Read the model definition and answer for the solid it produces. Units are mm, in the model's axes. Face numbers are marked on the shaded views. Coordinates: 2 decimals unless noted, no trailing zeros. Loops run counter-clockwise (first coordinate to the right, second up) from the corner with the lowest first, then second, coordinate; pieces in that order, holes last.
from build123d import *

# Parameters (mm, degrees)
SKETCH2_R               = 50
SKETCH2_R_2             = 25
BOSS_EXTRUDE1_DEPTH     = 10
CUT_EXTRUDE1_DEPTH      = 72.414284285
CUT_EXTRUDE1_DEPTH_BACK = 72.414284285
SKETCH3_R               = 1.5
SKETCH5_W               = 42.1
SKETCH5_H               = 42.1
SKETCH5_W_2             = 28.1
SKETCH5_H_2             = 28.1
BOSS_EXTRUDE3_DEPTH     = 32
SKETCH6_W               = 15
SKETCH6_H               = 10
CUT_EXTRUDE2_DEPTH      = 7
SKETCH7_W               = 42.1
SKETCH7_H               = 42.1
SKETCH7_R               = 14.05
BOSS_EXTRUDE4_DEPTH     = 40
CUT_EXTRUDE3_START      = -72
CUT_EXTRUDE3_DEPTH      = 72
CIRPATTERN1_COUNT       = 4
SKETCH12_R              = 21.05
SKETCH12_W              = 20.1
SKETCH12_H              = 20.1
BOSS_EXTRUDE5_DEPTH     = 10


with BuildPart() as part:
    # Sketch2 → Boss-Extrude1 (new body)
    with BuildSketch(Plane.XY):
        Circle(SKETCH2_R)
        Circle(SKETCH2_R_2, mode=Mode.SUBTRACT)
    extrude(amount=BOSS_EXTRUDE1_DEPTH)

    # Sketch3 → Cut-Extrude1 (cut, two sides: drawn at the far end of the back side and taken through both)
    with BuildSketch(Plane(origin=(0, 0, 0), x_dir=(1, 0, 0), z_dir=(0, 1, 0)).offset(-CUT_EXTRUDE1_DEPTH_BACK)):
        with Locations(Location((0, -5, 0), (0, 0, 270))):
            Circle(SKETCH3_R)
    extrude(amount=CUT_EXTRUDE1_DEPTH + CUT_EXTRUDE1_DEPTH_BACK, mode=Mode.SUBTRACT)



with BuildPart() as body_2:
    # Sketch5 → Boss-Extrude3 (new body)
    with BuildSketch(Plane.XY.offset(30)):
        Rectangle(SKETCH5_W, SKETCH5_H)
        Rectangle(SKETCH5_W_2, SKETCH5_H_2, mode=Mode.SUBTRACT)
    extrude(amount=BOSS_EXTRUDE3_DEPTH)

    # Sketch6 → Cut-Extrude2 (cut)
    with BuildSketch(Plane(origin=(0, 21.05, 0), x_dir=(1, 0, 0), z_dir=(0, 1, 0))):
        with Locations((0, -37.5)):
            Rectangle(SKETCH6_W, SKETCH6_H)
    extrude(amount=-CUT_EXTRUDE2_DEPTH, mode=Mode.SUBTRACT)

    # Sketch7 → Boss-Extrude4 (add)
    with BuildSketch(Plane.XY.offset(62)):
        Rectangle(SKETCH7_W, SKETCH7_H)
        Circle(SKETCH7_R, mode=Mode.SUBTRACT)
    extrude(amount=BOSS_EXTRUDE4_DEPTH)

    # Sketch11 → Cut-Extrude3 (cut)
    with BuildSketch(Plane.XY.offset(102).offset(CUT_EXTRUDE3_START)):
        with BuildLine():
            Line((0, 21.05), (-21.05, 21.05))
            Line((-21.05, 21.05), (-21.05, 0))
            ThreePointArc((-21.05, 0), (-14.884597744, 14.884597744), (0, 21.05))
        make_face()
    cut_extrude3 = extrude(amount=CUT_EXTRUDE3_DEPTH, mode=Mode.SUBTRACT)

    # CirPattern1: Cut-Extrude3 ×4 about axis
    cirpattern1_axis = Axis((0, 0, 102), (0, 0, 1))
    for i in range(1, CIRPATTERN1_COUNT):
        add(cut_extrude3.rotate(cirpattern1_axis, i * 360 / CIRPATTERN1_COUNT), mode=Mode.SUBTRACT)


with BuildPart() as part_1:
    add(part.part)

    add(body_2.part)  # Revolve2 merges body 2
    # Sketch10 → Revolve2 (revolve)
    with BuildSketch(Plane(origin=(0, 0, 0), x_dir=(1, 0, 0), z_dir=(0, 1, 0))):
        with BuildLine():
            Line((-50, -10), (-25, -10))
            add(Edge.make_bspline(
                [(-25, -10), (-21.924679616, -19.790318995), (-21.05, -30)],
                knots=[0, 0, 0, 1, 1, 1], degree=2))
            Line((-21.05, -30), (-21.05, -80))
            add(Edge.make_bspline(
                [(-50, -10), (-29.091325996, -42.246977979), (-21.05, -80)],
                knots=[0, 0, 0, 1, 1, 1], degree=2))
        make_face()
    revolve(axis=Axis((0, 0, 0), (0, 0, 1)))

    # Sketch12 → Boss-Extrude5 (add)
    with BuildSketch(Plane(origin=(0, 0, 30), x_dir=(-1, 0, 0), z_dir=(0, 0, -1))):
        with Locations(Location((0, 0, 0), (0, 0, 180))):
            Circle(SKETCH12_R)
        Rectangle(SKETCH12_W, SKETCH12_H, mode=Mode.SUBTRACT)
    extrude(amount=BOSS_EXTRUDE5_DEPTH)


solid = part_1.part
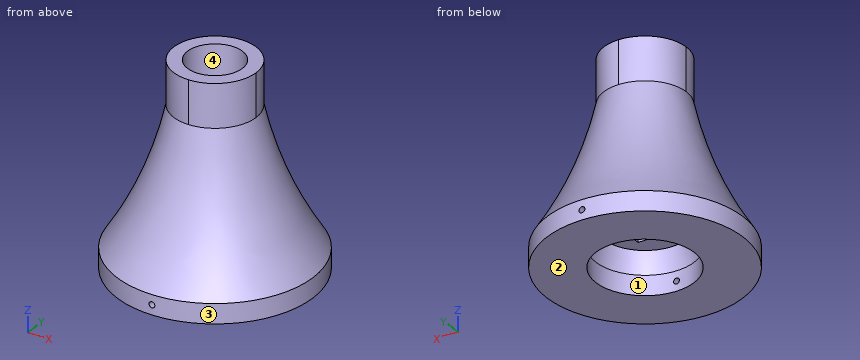
Item 1: Find the intervals of material crossed by line 1 along X through (y, z) = (0, 5); line 2 along Z through (x, y) = (7, -15.5), in increasing order.
Numbers:
line 1: x = -50 to -25, 25 to 50
line 2: z = 20 to 102
Item 2: A cutting plane is placed at A-A on z = 81.5. Determine the outline of the cut face in (x, y), then the cut area to 3 significant figures.
Numbers:
outline: circle Ø42.1 at (0, 0); hole circle Ø28.1 at (0, 0)
area: 772 mm2
Item 3: Given pin 1 (22.5 mm diameter, centred on y = 1.5, z = 40, fed in from +X); pin 2 (11 mm diameter, centred on x = 5, z = 25, fed in from -Y); pin 3 (3 mm diameter, centred on y = 1.5, z = 40, fed in from -X); pin 4 (8 mm diameter, centred on x = 37.5, y = 3.5, fed in from -Z), each flat-ended and moving along its own axis, determine where each tip first touches the part or whether it passes through.
Numbers:
pin 1: stops at x = 39.15
pin 2: stops at y = -43.95
pin 3: stops at x = -34.48
pin 4: stops at z = 0
Item 4: Determine the mould class of the marked faces 1, 2, 3 and 4 for opening direction X: released by +X, released by -X, zero draft, split by the parting line, or undercut.
Numbers:
face 1: undercut
face 2: zero draft
face 3: split by the parting line
face 4: undercut
